from build123d import *

# Parameters (mm, degrees)
SKETCH_1_W          = 47.5
SKETCH_1_H          = 60.8
EXTRUDE_1_DEPTH     = 30
SKETCH_3_W          = 37.5
SKETCH_3_H          = 45.8
CUT_EXTRUDE_1_DEPTH = 27
SKETCH_4_W          = 14
SKETCH_4_H          = 5
CUT_EXTRUDE_2_DEPTH = 8
SKETCH_5_R          = 3
SKETCH_5_W          = 6
SKETCH_5_H          = 6
EXTRUDE_4_DEPTH     = 20.5
SKETCH_6_W          = 5
SKETCH_6_H          = 10.5
EXTRUDE_6_DEPTH     = 25
SKETCH_7_R          = 1
EXTRUDE_7_DEPTH     = 3
SKETCH_12_W         = 5.3
SKETCH_12_H         = 4.5
CUT_EXTRUDE_5_DEPTH = 10
SKETCH_13_W         = 1.5
SKETCH_13_H         = 6
EXTRUDE_8_DEPTH     = 4.5
SKETCH_14_W         = 30
SKETCH_14_H         = 3
CUT_EXTRUDE_6_DEPTH = 3
CHAMFER_1_SIZE      = 1
SKETCH_16_W         = 12.5
SKETCH_16_H         = 4
SKETCH_16_W_2       = 7
SKETCH_16_H_2       = 2
EXTRUDE_9_DEPTH     = 5


with BuildPart() as part:
    # 草图1 → 凸台-拉伸1 (new body)
    with BuildSketch(Plane(origin=(0, 0, 0), x_dir=(1, 0, 0), z_dir=(0, 1, 0))):
        with Locations((-26.283333333, -1.583333333)):
            Rectangle(SKETCH_1_W, SKETCH_1_H)
    extrude(amount=EXTRUDE_1_DEPTH)

    # 草图3 → 切除-拉伸1 (cut)
    with BuildSketch(Plane(origin=(0, 30, 0), x_dir=(1, 0, 0), z_dir=(0, 1, 0))):
        with Locations((-26.283333333, -4.083333333)):
            Rectangle(SKETCH_3_W, SKETCH_3_H)
    extrude(amount=-CUT_EXTRUDE_1_DEPTH, mode=Mode.SUBTRACT)

    # 草图4 → 切除-拉伸2 (cut)
    with BuildSketch(Plane(origin=(0, 30, 0), x_dir=(1, 0, 0), z_dir=(0, 1, 0))):
        with Locations((-26.083333333, -29.483333333)):
            Rectangle(SKETCH_4_W, SKETCH_4_H)
    extrude(amount=-CUT_EXTRUDE_2_DEPTH, mode=Mode.SUBTRACT)

    # 草图5 → 凸台-拉伸4 (add)
    with BuildSketch(Plane(origin=(0, 3, 0), x_dir=(1, 0, 0), z_dir=(0, 1, 0))):
        with Locations(Location((-16.083333333, 4.816666667, 0), (0, 0, 270))):
            Circle(SKETCH_5_R)
        with Locations(Location((-36.483333333, 4.816666667, 0), (0, 0, 270))):
            Circle(SKETCH_5_R)
        with Locations((-25.533333333, -23.983333333)):
            Rectangle(SKETCH_5_W, SKETCH_5_H)
    extrude(amount=EXTRUDE_4_DEPTH)

    # 草图6 → 凸台-拉伸6 (add)
    with BuildSketch(Plane(origin=(0, 3, 0), x_dir=(1, 0, 0), z_dir=(0, 1, 0))):
        with Locations((-28.533333333, 13.566666667)):
            Rectangle(SKETCH_6_W, SKETCH_6_H)
    extrude(amount=EXTRUDE_6_DEPTH)

    # 草图7 → 凸台-拉伸7 (add)
    with BuildSketch(Plane(origin=(0, 23.5, 0), x_dir=(1, 0, 0), z_dir=(0, 1, 0))):
        with Locations(Location((-36.483333333, 4.816666667, 0), (0, 0, 270))):
            Circle(SKETCH_7_R)
        with Locations(Location((-16.083333333, 4.816666667, 0), (0, 0, 270))):
            Circle(SKETCH_7_R)
    extrude(amount=EXTRUDE_7_DEPTH)

    # 草图12 → 切除-拉伸5 (cut)
    with BuildSketch(Plane(origin=(0, 0, -28.816666667), x_dir=(-1, 0, 0), z_dir=(0, 0, -1))):
        with Locations((13.183333333, 27.75)):
            Rectangle(SKETCH_12_W, SKETCH_12_H)
    extrude(amount=-CUT_EXTRUDE_5_DEPTH, mode=Mode.SUBTRACT)

    # 草图13 → 凸台-拉伸8 (add)
    with BuildSketch(Plane(origin=(0, 25.5, 0), x_dir=(1, 0, 0), z_dir=(0, 1, 0))):
        with Locations((-13.183333333, 21.816666667)):
            Rectangle(SKETCH_13_W, SKETCH_13_H)
    extrude(amount=EXTRUDE_8_DEPTH)

    # 草图14 → 切除-拉伸6 (cut)
    with BuildSketch(Plane(origin=(0, 3, 0), x_dir=(1, 0, 0), z_dir=(0, 1, 0))):
        with Locations((-26.033333333, -2.090371048)):
            Rectangle(SKETCH_14_W, SKETCH_14_H)
        with Locations((-26.033333333, -8.090371048)):
            Rectangle(SKETCH_14_W, SKETCH_14_H)
        with Locations((-26.033333333, -14.090371048)):
            Rectangle(SKETCH_14_W, SKETCH_14_H)
    extrude(amount=-CUT_EXTRUDE_6_DEPTH, mode=Mode.SUBTRACT)

    # 倒角1
    chamfer_1_edges = [part.edges().sort_by_distance(p)[0] for p in [
        (-26.283333333, 0, -28.816666667),
        (-2.533333333, 0, 1.583333333),
        (-26.283333333, 0, 31.983333333),
        (-50.033333333, 0, 1.583333333),
        (-50.033333333, 15, -28.816666667),
        (-2.533333333, 15, -28.816666667),
        (-2.533333333, 15, 31.983333333),
        (-50.033333333, 15, 31.983333333),
    ]]
    chamfer(chamfer_1_edges, length=CHAMFER_1_SIZE)

    # 草图16 → 凸台-拉伸9 (add)
    with BuildSketch(Plane(origin=(0, 30, 0), x_dir=(1, 0, 0), z_dir=(0, 1, 0))):
        with Locations((-28.783333333, 23.816666667)):
            Rectangle(SKETCH_16_W, SKETCH_16_H)
        with Locations((-9.033333333, -29.483333333)):
            Rectangle(SKETCH_16_W_2, SKETCH_16_H_2)
        with Locations((-43.533333333, -29.483333333)):
            Rectangle(SKETCH_16_W_2, SKETCH_16_H_2)
    extrude(amount=EXTRUDE_9_DEPTH)


solid = part.part
Part model, mm, in its own coordinate system. A direction names the side the tool comes from. Coordinates: 2 decimals unless noted, no trailing zeros. Order: outer loops, then holes, each group sorted by start corner. A loop starts at its lowest first (then second) coordinate and runs counter-clockwise, first axis right, second up.
(1) Slice it at C-C, the plane z = -16.5. Write the cut outline in (x, y).
Check sheet entries:
outline: (-50.03, 1) - (-49.03, 0) - (-3.53, 0) - (-2.53, 1) - (-2.53, 30) - (-7.53, 30) - (-7.53, 3) - (-26.03, 3) - (-26.03, 28) - (-31.03, 28) - (-31.03, 3) - (-45.03, 3) - (-45.03, 30) - (-50.03, 30) - close
(2) Probe L1, parallel to X at y = 14, z = 24.5; L2, parallel to X at y = 23.5, z = -14; L3, parallel to X at y = 9, z = -4.5. List the from-to ranges inside material, lowest first.
Check sheet entries:
L1: x = -50.03 to -45.03, -28.53 to -22.53, -7.53 to -2.53
L2: x = -50.03 to -45.03, -31.03 to -26.03, -7.53 to -2.53
L3: x = -50.03 to -45.03, -39.47 to -33.5, -19.07 to -13.1, -7.53 to -2.53
(3) Tool access for faces 1 (the face through (-13.933, 28, -22)), 2 (the face through (-26, 23.5, 24)), 3 (the face through (-26, 13, 20.983)), 4 (the face through (-40.033, 32, 29)), 5 (the face through (-11.033, 2, 8)): list every direction of +Z, -Z, +X, -X, +Y, -Y with a clear straight run to the whole face (end or side of a thin tool).
Check sheet entries:
face 1: -Z, +Y
face 2: +Z, +Y
face 3: +Y
face 4: +Z, -Z, +Y
face 5: +Y, -Y
(4) Slice it at B-B, the plane y = 5. Write the cut outline in (x, z).
Check sheet entries:
outline: (-50.03, -27.82) - (-49.03, -28.82) - (-3.53, -28.82) - (-2.53, -27.82) - (-2.53, 30.98) - (-3.53, 31.98) - (-49.03, 31.98) - (-50.03, 30.98) - close; circle Ø6 at (-36.48, -4.82); circle Ø6 at (-16.08, -4.82); hole (-45.03, -18.82) - (-31.03, -18.82) - (-31.03, -8.32) - (-26.03, -8.32) - (-26.03, -18.82) - (-7.53, -18.82) - (-7.53, 26.98) - (-22.53, 26.98) - (-22.53, 20.98) - (-28.53, 20.98) - (-28.53, 26.98) - (-45.03, 26.98) - close
(5) Slice it at D-D, the plane z = 20. Write the cut outline in (x, y), and give its area (4 significant figures).
Check sheet entries:
outline: (-50.03, 1) - (-49.03, 0) - (-3.53, 0) - (-2.53, 1) - (-2.53, 30) - (-7.53, 30) - (-7.53, 3) - (-45.03, 3) - (-45.03, 30) - (-50.03, 30) - close
area: 411.5 mm2
(6) Pin check, flat tips, straight feed: pin 1 Ø5 at (x, z) = (-37.5, -3.5) entering from +Y; pin 2 Ø10 at (x, z) = (-26.5, 13) entering from +Y; pin 3 Ø1.5 at (x, y) = (-31.5, 31.5) entering from -Z. Stop position of each tip, or through.
Check sheet entries:
pin 1: stops at y = 26.5
pin 2: stops at y = 3
pin 3: stops at z = -25.82
(7) Slice it at A-A, the plane x = -29.5. Write the cut outline in (y, z), and give its area (3 significant figures).
Check sheet entries:
outline: (0, -27.82) - (1, -28.82) - (30, -28.82) - (30, -25.82) - (35, -25.82) - (35, -21.82) - (30, -21.82) - (30, -18.82) - (28, -18.82) - (28, -8.32) - (3, -8.32) - (3, 0.59) - (0, 0.59) - close; (0, 3.59) - (3, 3.59) - (3, 6.59) - (0, 6.59) - close; (0, 9.59) - (3, 9.59) - (3, 12.59) - (0, 12.59) - close; (0, 15.59) - (3, 15.59) - (3, 26.98) - (22, 26.98) - (22, 31.98) - (1, 31.98) - (0, 30.98) - close
area: 802 mm2
(8) Pull direction X, two halves, no side cores. Call faces 6 (the face through (-2.533, 15, 2)), 7 (the face through (-29, 32, -21.817)), 8 (the face through (-11.033, 2, 2)): pulls with the +X half, pulls with the -X half, needs draft (parallel to the pull), parting line crosses it, or undercut.
Check sheet entries:
face 6: pulls with the +X half
face 7: needs draft
face 8: undercut
